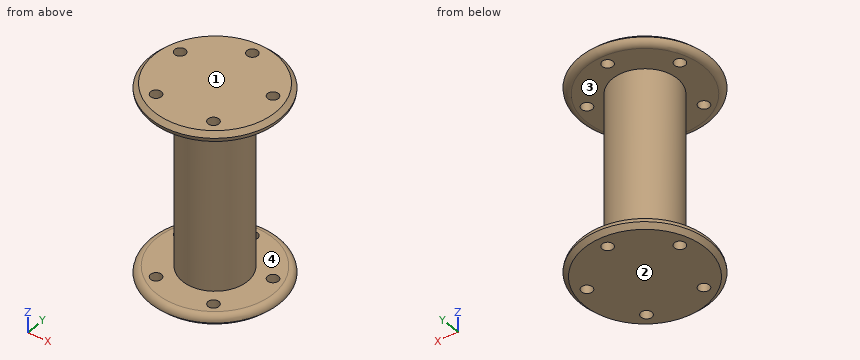
from build123d import *

# Parameters (mm, degrees)
SKETCH1_R                = 15
BOSS_EXTRUDE1_DEPTH      = 40
SKETCH2_R                = 30
BOSS_EXTRUDE2_DEPTH      = 5
CHAMFER1_SIZE            = 2
SKETCH5_R                = 2.5
CUT_EXTRUDE1_DEPTH       = 96
CIRPATTERN1_COUNT        = 5
FILLET1_R                = 3
MIRROR2_COPY_1_SKETCH_R  = 2.5
MIRROR2_COPY_1_DEPTH     = 96
MIRROR2_COPY_2_SKETCH_R  = 2.5
MIRROR2_COPY_2_DEPTH     = 96
MIRROR2_COPY_3_SKETCH_R  = 2.5
MIRROR2_COPY_3_DEPTH     = 96
MIRROR2_COPY_4_SKETCH_R  = 2.5
MIRROR2_COPY_4_DEPTH     = 96
CHAMFER1_OF_MIRROR2_SIZE = 2
FILLET1_OF_MIRROR2_R     = 3


with BuildPart() as part:
    # Sketch1 → Boss-Extrude1 (new, symmetric)
    with BuildSketch(Plane.XY):
        Circle(SKETCH1_R)
    extrude(amount=BOSS_EXTRUDE1_DEPTH, both=True)

    # Sketch2 → Boss-Extrude2 (add)
    with BuildSketch(Plane(origin=(0, 0, -40), x_dir=(-1, 0, 0), z_dir=(0, 0, -1))):
        Circle(SKETCH2_R)
    boss_extrude2 = extrude(amount=BOSS_EXTRUDE2_DEPTH)

    # Chamfer1
    chamfer1_edges = [part.edges().sort_by_distance(p)[0] for p in [
        (30, 0, -45),
    ]]
    chamfer(chamfer1_edges, length=CHAMFER1_SIZE)

    # Sketch5 → Cut-Extrude1 (cut, through all)
    with BuildSketch(Plane(origin=(0, 0, -45), x_dir=(-1, 0, 0), z_dir=(0, 0, -1))):
        with Locations((0, 22.5)):
            Circle(SKETCH5_R)
    cut_extrude1 = extrude(amount=-CUT_EXTRUDE1_DEPTH, mode=Mode.SUBTRACT)

    # CirPattern1: Cut-Extrude1 ×5 about axis
    cirpattern1_axis = Axis((0, 0, 0), (0, 0, 1))
    for i in range(1, CIRPATTERN1_COUNT):
        add(cut_extrude1.rotate(cirpattern1_axis, i * 360 / CIRPATTERN1_COUNT), mode=Mode.SUBTRACT)

    # Fillet1
    fillet1_edges = [part.edges().sort_by_distance(p)[0] for p in [
        (30, 0, -40),
    ]]
    fillet(fillet1_edges, radius=FILLET1_R - 0.0001)  # a hair under: the kernel refuses the full size

    # Mirror2: Boss-Extrude2, Cut-Extrude1 across plane
    add(boss_extrude2.mirror(Plane.XY))
    add(cut_extrude1.mirror(Plane.XY), mode=Mode.SUBTRACT)

    # Mirror2 copy 1 sketch → Mirror2 copy 1 (cut, through all)
    with BuildSketch(Plane(origin=(0, 0, 45), x_dir=(-0.30901699437494745, -0.9510565162951535, 0), z_dir=(0, 0, 1))):
        with Locations((0, -22.5)):
            Circle(MIRROR2_COPY_1_SKETCH_R)
    extrude(amount=-MIRROR2_COPY_1_DEPTH, mode=Mode.SUBTRACT)

    # Mirror2 copy 2 sketch → Mirror2 copy 2 (cut, through all)
    with BuildSketch(Plane(origin=(0, 0, 45), x_dir=(0.8090169943749473, -0.5877852522924732, 0), z_dir=(0, 0, 1))):
        with Locations((0, -22.5)):
            Circle(MIRROR2_COPY_2_SKETCH_R)
    extrude(amount=-MIRROR2_COPY_2_DEPTH, mode=Mode.SUBTRACT)

    # Mirror2 copy 3 sketch → Mirror2 copy 3 (cut, through all)
    with BuildSketch(Plane(origin=(0, 0, 45), x_dir=(0.8090169943749476, 0.587785252292473, 0), z_dir=(0, 0, 1))):
        with Locations((0, -22.5)):
            Circle(MIRROR2_COPY_3_SKETCH_R)
    extrude(amount=-MIRROR2_COPY_3_DEPTH, mode=Mode.SUBTRACT)

    # Mirror2 copy 4 sketch → Mirror2 copy 4 (cut, through all)
    with BuildSketch(Plane(origin=(0, 0, 45), x_dir=(-0.30901699437494723, 0.9510565162951536, 0), z_dir=(0, 0, 1))):
        with Locations((0, -22.5)):
            Circle(MIRROR2_COPY_4_SKETCH_R)
    extrude(amount=-MIRROR2_COPY_4_DEPTH, mode=Mode.SUBTRACT)

    # Chamfer1 of Mirror2
    chamfer1_of_mirror2_edges = [part.edges().sort_by_distance(p)[0] for p in [
        (30, 0, 45),
    ]]
    chamfer(chamfer1_of_mirror2_edges, length=CHAMFER1_OF_MIRROR2_SIZE)

    # Fillet1 of Mirror2
    fillet1_of_mirror2_edges = [part.edges().sort_by_distance(p)[0] for p in [
        (30, 0, 40),
    ]]
    fillet(fillet1_of_mirror2_edges, radius=FILLET1_OF_MIRROR2_R - 0.0001)  # a hair under: the kernel refuses the full size


solid = part.part
Part model, mm, in its own coordinate system. Face numbers are marked on the shaded views. Coordinates: 2 decimals unless noted, no trailing zeros. Write each loop counter-clockwise with the first axis right and the second up, starting at its lowest first coordinate (ties: lowest second). Pieces come first, ordered by that corner, then holes. Notation, with made-up numbers: M 13,14.25 L 23,14.25 A22 ccw 23,47.25 Z; hole C -6.75,9 d1. An arc over 180 degrees is marked long. Return JSON: item names as keys, results as strings.
1. Probe L1, parallel to Z at x = -8, y = -17.5; L2, parallel to Y at x = 0, z = 43.25; L3, parallel to Y at x = 11, z = 32. List the from-to ranges inside material, lowest first.
Determined:
{"L1": "-45 to -40, 40 to 45", "L2": "-29.75 to 20, 25 to 29.75", "L3": "-10.2 to 10.2"}
2. Saw through at C-C, the plane z = 6.5. Write the cut outline in (x, y).
Determined:
{"outline": "C 0,0 d30"}
3. Flat gauge pins, fed straight in: pin 1 Ø12 at (y, z) = (16.5, 25) entering from +X; pin 2 Ø3 at (x, z) = (12, 25) entering from -Y; pin 3 Ø1 at (y, z) = (6.5, -16) entering from -X. Where does each tip first touch, or does it go through?
Determined:
{"pin 1": "x = 10.71", "pin 2": "y = -10.71", "pin 3": "x = -13.75"}
4. Saw through at A-A, the plane x = 0. Count the separate pieces of the cut face and the enclosed holes in it, then the cut area to 3 significant figures.
Determined:
{"separate pieces": "3", "enclosed holes": "0", "area": "2,930 mm²"}
5. Pull direction Z, two halves, no side cores. Call the marked faces 1, 2, 3 and 4: pulls with the +Z half, pulls with the -Z half, needs draft (parallel to the pull), parting line crosses it, or undercut.
Determined:
{"face 1": "pulls with the +Z half", "face 2": "pulls with the -Z half", "face 3": "undercut", "face 4": "undercut"}
